The model under review builds one solid part; all positions refer to its coordinate system, in mm. A direction names the side the tool comes from. Coordinates: 2 decimals unless noted, no trailing zeros. Order: outer loops, then holes, each group sorted by start corner. A loop starts at its lowest first (then second) coordinate and runs counter-clockwise, first axis right, second up. Notation, with made-up numbers: (19.25, 75) -> (66.25, 75) arc R21 cw to (66.25, 113) -> close; hole circle Ø3 at (29, 14.5). An arc over 180 degrees is marked (long way). Use CSV: the item, a comma, the result in double quotes. Start each with the question number.
```python
from build123d import *

# Parameters (mm, degrees)
SKETCH099_W             = 39.2
SKETCH099_H             = 8.4
SKETCH099_W_2           = 7.2
SKETCH099_H_2           = 7.2
SKETCH099_W_3           = 20
SKETCH099_H_3           = 7
PAD061_DEPTH            = 8
CYLINDER082_R           = 4
CYLINDER082_DEPTH       = 5
BOX007_W                = 3
BOX007_H                = 1
BOX007_DEPTH            = 8
CYLINDER083_R           = 2.4
CYLINDER083_DEPTH       = 10
BODY094_PLACEMENT_ANGLE = 90


with BuildPart() as part:
    # Sketch099 → Pad061 (new body)
    with BuildSketch(Plane.XY):
        Rectangle(SKETCH099_W, SKETCH099_H)
        with Locations((-15, 0)):
            Rectangle(SKETCH099_W_2, SKETCH099_H_2, mode=Mode.SUBTRACT)
        with Locations((15, 0)):
            Rectangle(SKETCH099_W_2, SKETCH099_H_2, mode=Mode.SUBTRACT)
        Rectangle(SKETCH099_W_3, SKETCH099_H_3, mode=Mode.SUBTRACT)
    extrude(amount=PAD061_DEPTH)

    # Cylinder082 → Cylinder082 (cut)
    with BuildSketch(Plane(origin=(0, 0, 8), x_dir=(1, 0, 0), z_dir=(0, -1, 0))):
        Circle(CYLINDER082_R)
    cylinder082 = extrude(amount=CYLINDER082_DEPTH, mode=Mode.SUBTRACT)

    # Mirrored017: Cylinder082 across XZ
    add(cylinder082.mirror(Plane.XZ), mode=Mode.SUBTRACT)

    # Box007 → Box007 (join)
    with BuildSketch(Plane(origin=(-16.5, 4, 0), x_dir=(1, 0, 0), z_dir=(0, -1, 0))):
        with Locations((1.5, 0.5)):
            Rectangle(BOX007_W, BOX007_H)
    box007 = extrude(amount=BOX007_DEPTH)

    # Mirrored018: Box007 across YZ
    add(box007.mirror(Plane.YZ))

    # Cylinder083 → Cylinder083 (cut)
    with BuildSketch(Plane(origin=(-7.25, 5, 4), x_dir=(1, 0, 0), z_dir=(0, -1, 0))):
        Circle(CYLINDER083_R)
    cylinder083 = extrude(amount=CYLINDER083_DEPTH, mode=Mode.SUBTRACT)

    # Mirrored019: Cylinder083 across YZ
    add(cylinder083.mirror(Plane.YZ), mode=Mode.SUBTRACT)


with BuildPart() as part_1:
    # Body088 placement: moved
    add(part.part.moved(Location((0, 0, -10.5))))


with BuildPart() as part_2:
    # Body094 placement: moved
    add(part_1.part.moved(Location((40, 17, 54))).rotate(Axis((40, 17, 54), (-1, 0, 0)), BODY094_PLACEMENT_ANGLE))


solid = part_2.part
```
Q1. Clearance check with flat-ended pins moving along their axes: pin 1 Ø2 at (x, z) = (43.5, 52) entering from +Y; pin 2 Ø2.5 at (x, z) = (25.5, 52.5) entering from +Y. State where each tip first meets the part, or that it passes through.
Q2. Add section D-D, the plane x = 54. State the section outline as (y, z) points.
Q3. Add section A-A, the plane x = 47.25. State the section outline as (y, z) points, then the cut area to 3 significant figures.
Q4. Add section B-B, the plane z = 53.5. State the section outline as (x, y) points.
Q5. Draft analysis for pull direction X (two halves, no side actions). For faces 4 (the flat face through (20.4, 10, 54)), 5 (the flat face through (55, 10, 57.6)), 6 (the flat face through (40, 10, 58.2)), state which applies: +X half, -X half, draft (parallel to the pull), parting line (faces both ways), or undercut.
Q6. For faces 1 (the flat face through (40, 10, 50.5)), 2 (the flat face through (29.8, 14.5, 53.9)), 3 (the flat face through (55, 7.5, 54)), list the 3-axis set-ups (+Z, -Z, +X, -X, +Y, -Y) from which the entire face can be reached by the end or side of a thin tool; tool diameter is ignored.
Q7. To check wall thickness, follow probe 1 along X at (y, z) = (14, 51.25); probe 2 along X at (y, z) = (7, 52.75); probe 3 along Z at (x, y) = (56, 11.25). State the ranges of each line that lie inside material, in increasing order.
Q8. Add section C-C, the plane x = 40. State the section outline as (y, z) points.
Answer block:
1,pin 1,"passes through"
1,pin 2,"stops at y = 7.5"
2,outline,"(6.5, 49.8) -> (14.5, 49.8) -> (14.5, 50.4) -> (7.5, 50.4) -> (7.5, 57.6) -> (14.5, 57.6) -> (14.5, 58.2) -> (6.5, 58.2) -> close"
3,outline,"(6.5, 49.8) -> (8.1, 49.8) -> (8.1, 50.5) -> (6.5, 50.5) -> close; (6.5, 57.5) -> (8.1, 57.5) -> (8.1, 58.2) -> (6.5, 58.2) -> close; (12.9, 49.8) -> (14.5, 49.8) -> (14.5, 50.5) -> (12.9, 50.5) -> close; (12.9, 57.5) -> (14.5, 57.5) -> (14.5, 58.2) -> (12.9, 58.2) -> close"
3,area,"4.48 mm²"
4,outline,"(20.4, 6.5) -> (21.4, 6.5) -> (21.4, 14.5) -> (20.4, 14.5) -> close; (23.5, 6.5) -> (26.5, 6.5) -> (26.5, 7.5) -> (23.5, 7.5) -> close; (28.6, 6.5) -> (30, 6.5) -> (30, 14.5) -> (28.6, 14.5) -> close; (50, 6.5) -> (51.4, 6.5) -> (51.4, 14.5) -> (50, 14.5) -> close; (53.5, 6.5) -> (56.5, 6.5) -> (56.5, 7.5) -> (53.5, 7.5) -> close; (58.6, 6.5) -> (59.6, 6.5) -> (59.6, 14.5) -> (58.6, 14.5) -> close"
5,face 4,"-X half"
5,face 5,"undercut"
5,face 6,"draft"
6,face 1,"+Y, -Y"
6,face 2,"+Z, -Z, +X, -X, +Y"
6,face 3,"+Y"
7,probe 1,"x = 20.4 to 21.4, 28.6 to 30, 50 to 51.4, 58.6 to 59.6"
7,probe 2,"x = 20.4 to 21.4, 23.5 to 26.5, 28.6 to 30, 50 to 51.4, 53.5 to 56.5, 58.6 to 59.6"
7,probe 3,"z = 49.8 to 50.4, 57.6 to 58.2"
8,outline,"(6.5, 49.8) -> (10.5, 49.8) -> (10.5, 50.5) -> (6.5, 50.5) -> close; (6.5, 57.5) -> (10.5, 57.5) -> (10.5, 58.2) -> (6.5, 58.2) -> close"
